Verification items for the finished model (mm, model axes). Face numbers are marked on the shaded views. A direction names the side the tool comes from. Round coordinates to 2 decimals unless told otherwise and drop trailing zeros. Loops run counter-clockwise (first coordinate to the right, second up) from the corner with the lowest first, then second, coordinate; pieces in that order, holes last. Notation, with made-up numbers: M 26,24 L 53,24 A21 ccw 53,40 Z; hole C -38,-15 d7. An arc over 180 degrees is marked long. Write item = value, one per line. Start each with the question number.
Autodesk Inventor part; units mm, degrees
ref_plane "body_to_B_L__XY" through (0, 0, 0) normal (1, 0, 0) x (0, 0, -1)
ref_plane "body_to_B_L__YZ" through (0, 0, 0) normal (0, 0, -1) x (0, 1, 0)
ref_plane "body_to_B_L__ZX" through (0, 0, 0) normal (0, 1, 0) x (1, 0, 0)
sketch "Sketch_1" plane through (0, 0, 0) normal (0, 0, 1) x (1, 0, 0)
  line L0 (30, 0) -> (0, 0)
  line L1 (0, 7.5) -> (5, 7.5)
  line L2 (5, 7.5) -> (5, 5)
  line L3 (5, 5) -> (25, 5)
  line L4 (25, 5) -> (25, 7.5)
  line L5 (25, 7.5) -> (30, 7.5)
  line L6 (30, 7.5) -> (30, 10)
  line L7 (30, 10) -> (0, 10)
  line L8 (0, 10) -> (0, 7.5)
revolve "Revolution1" add sketch "Sketch_1" angle 360 about axis through (30, 0, 0) along (1, 0, 0)
ref_plane "body_to_B_L__XY" through (0, 0, 0) normal (1, 0, 0) x (0, 0, -1)
ref_plane "body_to_B_L__YZ" through (0, 0, 0) normal (0, 0, -1) x (0, 1, 0)
ref_plane "body_to_B_L__ZX" through (0, 0, 0) normal (0, 1, 0) x (1, 0, 0)
ref_plane "body_to_B_R__XY" through (25, 0, 0) normal (-1, 0, 0) x (0, 0, -1)
ref_plane "body_to_B_R__YZ" through (25, 0, 0) normal (0, 0, -1) x (0, -1, 0)
ref_plane "body_to_B_R__ZX" through (25, 0, 0) normal (0, -1, 0) x (-1, 0, 0)
properties part number "RORPOS20-L30_1"
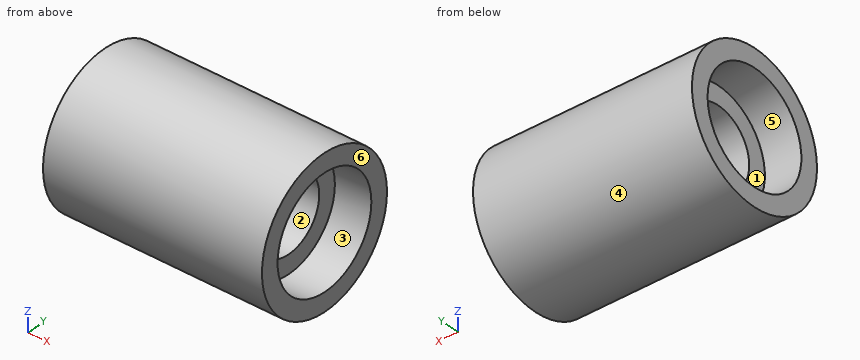
1. Section check A-A, the plane y = 0. Enter the section's corners in (x, z).
2. Section check D-D, the plane y = -8. Enter the section's corners in (x, z), and give its area (3 significant figures).
3. Tool access check on the marked faces 1, 2 and 3. Record the directions out of +Z, -Z, +X, -X, +Y, -Y that give a thin tool (end or side, any length) a straight path to the whole face; none if there is none.
4. Mould release check, pull along Z, two halves, no side actions. Record for the marked faces 4, 5 and 6: pulls with the +Z half, pulls with the -Z half, needs draft (parallel to the pull), parting line crosses it, or undercut.
5. Gauge pin test, flat ends, axial feed: P1, Ø3, axis at x = 25.5, z = 5.5, coming from the -Y side; P2, Ø5, axis at y = 1, z = 0.5, coming from the -X side; P3, Ø1.5, axis at x = 11, z = 4, coming from the -Y side; P4, Ø6, axis at y = 1.5, z = 6, coming from the -X side. Record the tip position at first contact, or that the pin passes through.
6. Section check C-C, the plane x = 25.75. Enter the section's corners in (y, z).
7. Thickness scan on line 1 (Z direction, x = 2.8, y = 0); line 2 (Z direction, x = 12.75, y = 0.25); line 3 (Y direction, x = 19.5, z = 2.5). Record the ranges inside material, lowest first.
Computed values:
q1.outline = M 0,-10 L 30,-10 L 30,-7.5 L 25,-7.5 L 25,-5 L 5,-5 L 5,-7.5 L 0,-7.5 Z; M 0,7.5 L 5,7.5 L 5,5 L 25,5 L 25,7.5 L 30,7.5 L 30,10 L 0,10 Z
q2.outline = M 0,-6 L 30,-6 L 30,6 L 0,6 Z
q2.area = 360 mm2
q3.face_1 = -X
q3.face_2 = +X, -X
q3.face_3 = +X
q4.face_4 = parting line crosses it
q4.face_5 = undercut
q4.face_6 = needs draft
q5.P1 = -9.17
q5.P2 = through
q5.P3 = -9.46
q5.P4 = 0
q6.outline = C 0,0 d20; hole C 0,0 d15
q7.line_1 = -10 to -7.5, 7.5 to 10
q7.line_2 = -10 to -4.99, 4.99 to 10
q7.line_3 = -9.68 to -4.33, 4.33 to 9.68
